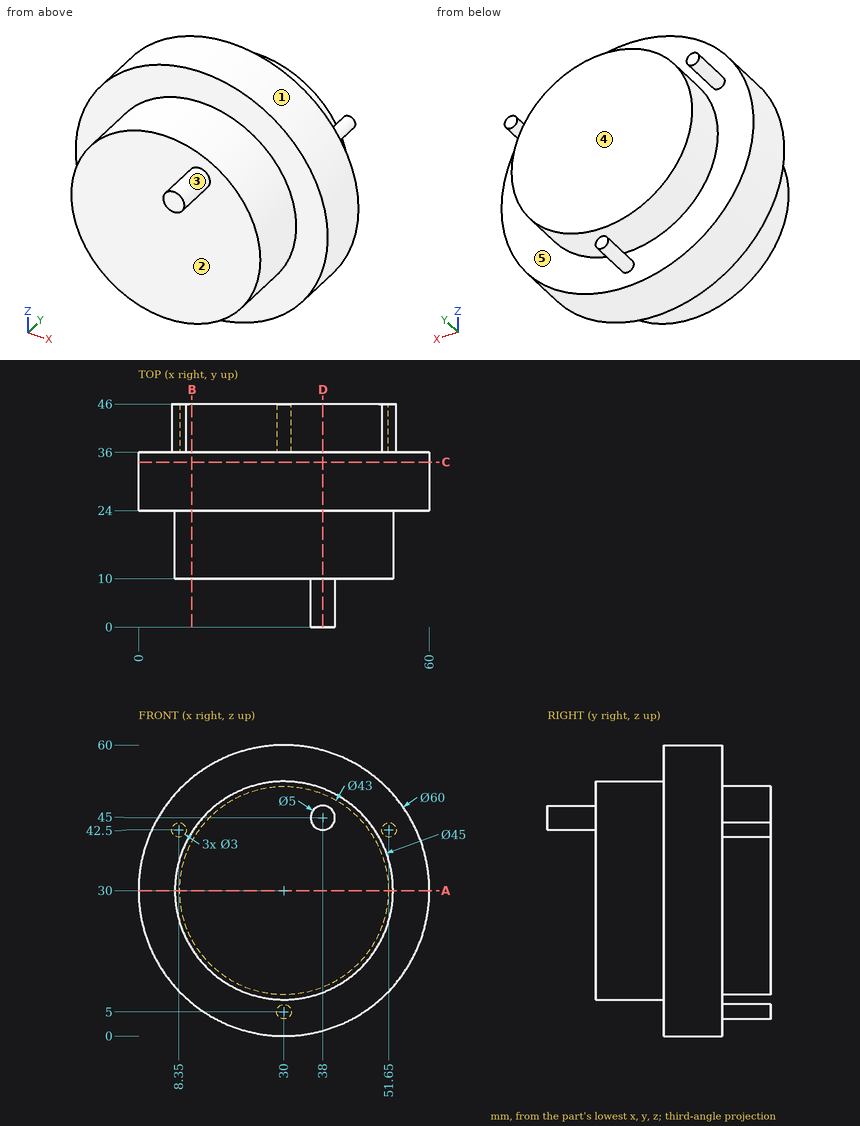
Design review of the part shown in the three views and the two pictorial views. Dimensions are in mm from the part's minimum x, y and z. A direction names the side the tool comes from. Round coordinates to 2 decimals unless told otherwise and drop trailing zeros. Loops run counter-clockwise (first coordinate to the right, second up) from the corner with the lowest first, then second, coordinate; pieces in that order, holes last. Notation, with made-up numbers: (-39.75, -40) - (-11.75, -40) arc R13 ccw to (-11.75, -23) - close; hole circle Ø7 at (34.5, -21.5). An arc over 180 degrees is marked (long way). One line per item, written item: value. Start each with the question number.
Item 1: Take a section at B-B (x = 11). Give the boundary of the cut face in (y, z), plus the area to 3 significant figures.
Item 2: For the marked faces 3, 4 and 5, list the 3-axis set-ups (+Z, -Z, +X, -X, +Y, -Y) from which the entire face can be reached by the end or side of a thin tool; tool diameter is ignored.
Item 3: Take a section at D-D (x = 38). Give the boundary of the cut face in (y, z).
Item 4: Take a section at C-C (y = 34). Give the boundary of the cut face in (x, z), plus the area to 3 significant figures.
Item 5: The part is to be moulded in two halves that separate along Z. For the marked faces 1 and 2, say which applies: +Z half, -Z half, draft (parallel to the pull), parting line (faces both ways), or undercut.
Item 6: Clearance check with flat-ended pins moving along their axes: pin 1 Ø6 at (x, z) = (39.5, 36.5) entering from -Y; pin 2 Ø8 at (y, z) = (19.5, 12) entering from +X; pin 3 Ø8 at (y, z) = (31, 12.5) entering from -X. State where each tip first meets the part, or that it passes through.
Item 7: Take a section at A-A (z = 30). Give the boundary of the cut face in (x, y), plus the area to 3 significant figures.
Item 8: For L1, parallel to Y at x = 26, z = 27; L2, parallel to Y at x = 39, z = 52; L3, parallel to X at y = 29, z = 30.5, list the stretches that pass through material, from the lowest coordinate up.
Answer below:
1. outline: (10, 17.95) - (24, 17.95) - (24, 6.78) - (36, 6.78) - (36, 19.94) - (46, 19.94) - (46, 40.06) - (36, 40.06) - (36, 53.22) - (24, 53.22) - (24, 42.05) - (10, 42.05) - close
1. area: 1,100 mm2
2. face 3: -Y
2. face 4: +Z, -Z, +X, -X, +Y
2. face 5: +Y
3. outline: (0, 42.5) - (10, 42.5) - (10, 8.97) - (24, 8.97) - (24, 1.09) - (36, 1.09) - (36, 10.04) - (46, 10.04) - (46, 49.96) - (36, 49.96) - (36, 58.91) - (24, 58.91) - (24, 51.03) - (10, 51.03) - (10, 47.5) - (0, 47.5) - close
4. outline: circle Ø60 at (30, 30)
4. area: 2,830 mm2
5. face 1: parting line
5. face 2: draft
6. pin 1: stops at y = 10
6. pin 2: stops at x = 47.61
6. pin 3: stops at x = 3.21
7. outline: (0, 24) - (7.5, 24) - (7.5, 10) - (52.5, 10) - (52.5, 24) - (60, 24) - (60, 36) - (51.5, 36) - (51.5, 46) - (8.5, 46) - (8.5, 36) - (0, 36) - close
7. area: 1,780 mm2
8. L1: y = 10 to 46
8. L2: y = 24 to 36
8. L3: x = 0 to 60
